The drawing under review shows one solid part. Ordinate dimensions are in mm from its lowest x, y, z. A direction names the side the tool comes from. Give positions to 0.01 mm unless a question says otherwise; leave off trailing zeros. Order: outer loops, then holes, each group sorted by start corner. A loop starts at its lowest first (then second) coordinate and runs counter-clockwise, first axis right, second up. Notation, with made-up numbers: (40.5, -13) -> (81.5, -13) arc R24 ccw to (81.5, 25) -> close; hole circle Ø9 at (82.25, 44.5). An arc over 180 degrees is marked (long way). One line per item, written item: value.
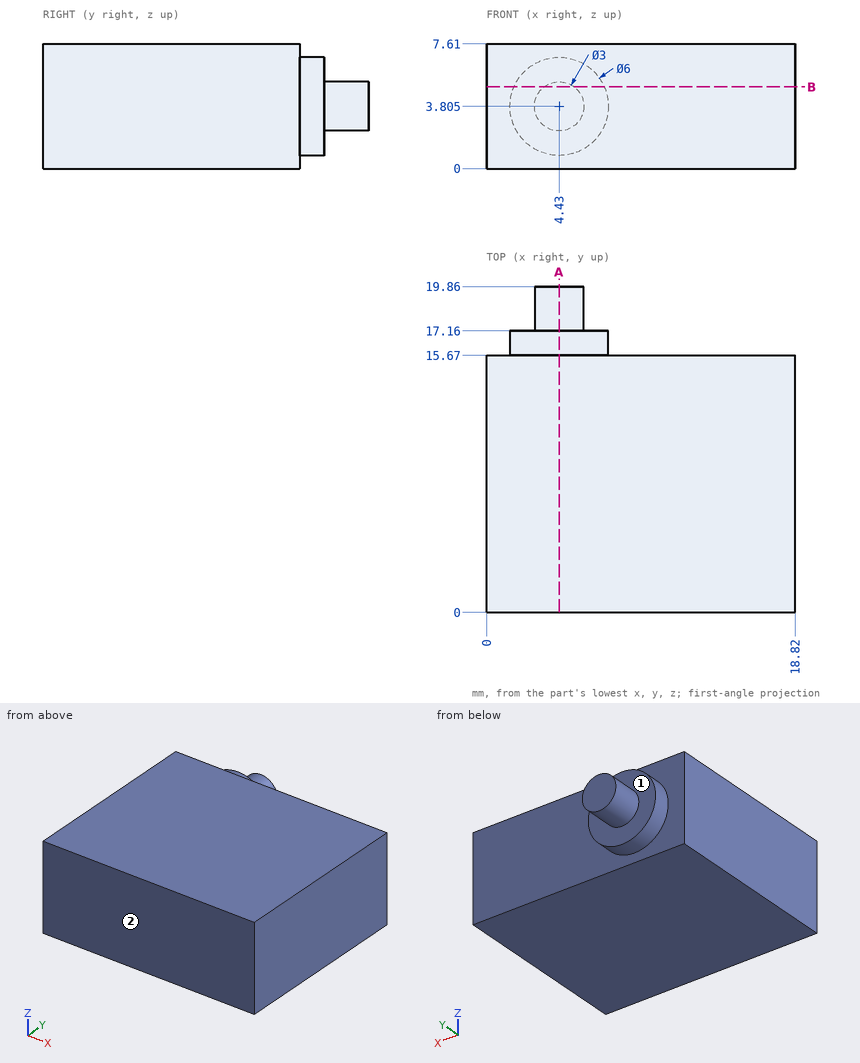
Item 1: Clearance check with flat-ended pins moving along their axes: P1, Ø4, axis at x = 8, z = 2, coming from the +Y side; P2, Ø2, axis at x = 9.5, z = 5.5, coming from the +Y side. State where each tip first meets the part, or that it passes through.
Returned:
P1: y = 17.16
P2: y = 15.67
Item 2: Add section A-A on x = 4.43. Give the boundary of the cut face in (y, z) (3 decimals).
Returned:
outline: (0, 0) -> (15.67, 0) -> (15.67, 0.805) -> (17.16, 0.805) -> (17.16, 2.305) -> (19.86, 2.305) -> (19.86, 5.305) -> (17.16, 5.305) -> (17.16, 6.805) -> (15.67, 6.805) -> (15.67, 7.61) -> (0, 7.61) -> close
Item 3: Add section B-B on z = 5. Give the boundary of the cut face in (x, y).
Returned:
outline: (0, 0) -> (18.82, 0) -> (18.82, 15.67) -> (7.18, 15.67) -> (7.18, 17.16) -> (5.34, 17.16) -> (5.34, 19.86) -> (3.52, 19.86) -> (3.52, 17.16) -> (1.68, 17.16) -> (1.68, 15.67) -> (0, 15.67) -> close
Item 4: To check wall thickness, follow line 1 along Y through (x, z) = (14.5, 4.75); line 2 along Y through (x, z) = (3, 3.25); line 3 along Z through (x, y) = (5.5, 17.75). State the ranges of each line that lie inside material, in increasing order. Write a range as from..to.
Returned:
line 1: 0..15.67
line 2: 0..17.16
line 3: 2.75..4.86
Item 5: Machinability: for the marked faces 1 and 2, which of the approach directions +Z, -Z, +X, -X, +Y, -Y give a long, thin tool a straight path to every point of the face, cutting with its end or side? Answer none if there is none.
Returned:
face 1: +Y
face 2: +Z, -Z, +X, -X, -Y
